Work out the finished part from the listing and answer in its coordinate system (mm). A direction names the side the tool comes from. Coordinates: 2 decimals unless noted, no trailing zeros. Write each loop counter-clockwise with the first axis right and the second up, starting at its lowest first coordinate (ties: lowest second). Pieces come first, ordered by that corner, then holes. Notation, with made-up numbers: (29, 87.5) - (76, 87.5) arc R27 cw to (76, 120.5) - close; hole circle Ø9 at (81, -21.5). An arc over 180 degrees is marked (long way). One line per item, written item: value.
Autodesk Inventor part; units mm, degrees
ref_plane "YZ Plane" through (0, 0, 0) normal (1, 0, 0) x (0, 1, 0)
ref_plane "XZ Plane" through (0, 0, 0) normal (0, 1, 0) x (-1, 0, 0)
ref_plane "XY Plane" through (0, 0, 0) normal (0, 0, 1) x (1, 0, 0)
sketch "Sketch1" plane through (0, 0, 0) normal (0, 1, 0) x (-1, 0, 0)
  line L0 (0, 5) -> (0, 5)
  line L1 (-2, 3) -> (-2, -3)
  line L2 (0, -5) -> (0, -5)
  line L3 (2, -3) -> (2, 3)
  line L4 (2, 5) -> (-2, -5) construction
  line L5 (-2, 5) -> (2, -5) construction
  arc A0 (2, 3) -> (0, 5) centre (0, 3) ccw
  arc A1 (0, -5) -> (2, -3) centre (0, -3) ccw
  arc A2 (-2, -3) -> (0, -5) centre (0, -3) ccw
  arc A3 (0, 5) -> (-2, 3) centre (0, 3) ccw
  line L6 (1.25, 0.6) -> (-1.25, 0.6)
  line L7 (-1.25, 0.6) -> (-1.25, -0.6)
  line L8 (-1.25, -0.6) -> (1.25, -0.6)
  line L9 (1.25, -0.6) -> (1.25, 0.6)
  line L10 (1.25, 0.6) -> (-1.25, -0.6) construction
  line L11 (-1.25, 0.6) -> (1.25, -0.6) construction
  arc A4 (-1.25, -2.1) -> (1.25, -2.1) centre (0, -1.6) ccw
  line L12 (-1.25, -2.1) -> (1.25, -2.1)
  line L13 (2, 0) -> (-2.9121, 0) construction
  arc A5 (1.25, 2.1) -> (-1.25, 2.1) centre (0, 1.6) ccw
  line L14 (-1.25, 2.1) -> (1.25, 2.1)
  point P0 (0, 0)
  dimension "d0" = 10
  dimension "d1" = 4
  dimension "d2" = 2
  dimension "d3" = 1.2
  dimension "d4" = 2.5
  dimension "d5" = 1.5
  dimension "d6" = 1.5
  dimension "d7" = 1
  dimension "d8" = 1.3463
  dimension "d9" = 0.75
extrude "Extrusion1" add sketch "Sketch1" along normal blind 10
properties part number "Pressure sensor connector" material "PET Plastic"
Item 1: Section D-D, the plane z = 4 is taken. Determine the outline of the cut face in (x, y), then the cut area to 3 significant figures.
Evaluation:
outline: (-1.73, 0) - (1.73, 0) - (1.73, 10) - (-1.73, 10) - close
area: 34.6 mm2
Item 2: Determine the mould class of faces 3 (the face through (2, 5, 0)), 4 (the face through (0, 5, 0.6)), 5 (the face through (0, 5, -5)) for opening direction Z: +Z half, -Z half, draft (parallel to the pull), parting line (faces both ways), or undercut.
Evaluation:
face 3: draft
face 4: undercut
face 5: -Z half
Item 3: Consider probe 1 along Z at (x, y) = (0.1, 5); probe 2 along X at (y, z) = (6.25, -0.25); probe 3 along Z at (x, y) = (-0.5, 9.5). Determine where each line is inside the solid, lowest interval first.
Evaluation:
probe 1: z = -5 to -2.94, -2.1 to -0.6, 0.6 to 2.1, 2.94 to 5
probe 2: x = -2 to -1.25, 1.25 to 2
probe 3: z = -4.94 to -2.85, -2.1 to -0.6, 0.6 to 2.1, 2.85 to 4.94
Item 4: Given pin 1 (0.8 mm diameter, centred on x = -0.5, y = 4, fed in from +Z), flat-ended and moving along its own axis, determine where the tip first touches the part or whether it passes through.
Evaluation:
pin 1: stops at z = 5
Item 5: Section C-C, the plane y = 2.5 is taken. Determine the outline of the cut face in (x, z), then the cut area to 3 significant figures.
Evaluation:
outline: (-2, -3) arc R2 ccw to (2, -3) - (2, 3) arc R2 ccw to (-2, 3) - close; hole (-1.25, -2.1) arc R1.35 ccw to (1.25, -2.1) - close; hole (-1.25, -0.6) - (1.25, -0.6) - (1.25, 0.6) - (-1.25, 0.6) - close; hole (-1.25, 2.1) - (1.25, 2.1) arc R1.35 ccw to start
area: 30.5 mm2
Item 6: Which of the six approach directions +Z, -Z, +X, -X, +Y, -Y give full straight-line access (tool end or side, diameter ignored) to faces 1 (the face through (0, 10, -1)), 2 (the face through (0, 5, -0.6))?
Evaluation:
face 1: +Z, -Z, +X, -X, +Y
face 2: +Y, -Y
Item 7: Section B-B, the plane z = -2.5 is taken. Determine the outline of the cut face in (x, y), then the cut area to 3 significant figures.
Evaluation:
outline: (-2, 0) - (-1, 0) - (-1, 10) - (-2, 10) - close; (1, 0) - (2, 0) - (2, 10) - (1, 10) - close
area: 20.0 mm2
Item 8: Section A-A, the plane x = 0 is taken. Determine the outline of the cut face in (y, z), then the cut area to 3 significant figures.
Evaluation:
outline: (0, -5) - (10, -5) - (10, -2.95) - (0, -2.95) - close; (0, -2.1) - (10, -2.1) - (10, -0.6) - (0, -0.6) - close; (0, 0.6) - (10, 0.6) - (10, 2.1) - (0, 2.1) - close; (0, 2.95) - (10, 2.95) - (10, 5) - (0, 5) - close
area: 71.1 mm2
